from build123d import *

# Parameters (mm, degrees)
SKETCH1_W            = 40
SKETCH1_H            = 15
BOSS_EXTRUDE1_DEPTH  = 6
M3_CLEARANCE_HOLE1_D = 3.2
FILLET1_R            = 5


with BuildPart() as part:
    # Sketch1 → Boss-Extrude1 (new body)
    with BuildSketch(Plane(origin=(0, 0, 0), x_dir=(1, 0, 0), z_dir=(0, 1, 0))):
        Rectangle(SKETCH1_W, SKETCH1_H)
    extrude(amount=BOSS_EXTRUDE1_DEPTH)

    # M3 Clearance Hole1 (through all)
    with Locations(Plane(origin=(0, 6, 0), x_dir=(1, 0, 0), z_dir=(0, 1, 0))):
        with Locations((-15, 0), (15, 0)):
            Hole(M3_CLEARANCE_HOLE1_D / 2)

    # Fillet1
    fillet1_edges = [part.edges().sort_by_distance(p)[0] for p in [
        (20, 3, 7.5),
        (-20, 3, 7.5),
        (-20, 3, -7.5),
        (20, 3, -7.5),
    ]]
    fillet(fillet1_edges, radius=FILLET1_R)


solid = part.part
Verification items for the finished model (mm, model axes). Round coordinates to 2 decimals unless told otherwise and drop trailing zeros. Loops run counter-clockwise (first coordinate to the right, second up) from the corner with the lowest first, then second, coordinate; pieces in that order, holes last. Notation, with made-up numbers: (34, 11.5) - (66, 11.5) arc R9 cw to (66, 20.5) - close; hole circle Ø11 at (76, -31.5). An arc over 180 degrees is marked (long way). Use a Markdown table: item, result. Add a question column.
1. Gauge pin test, flat end, axial feed: pin 1 (1.5 mm diameter, centred on y = 4.5, z = -5.5, fed in from +X). Record the tip position at first contact, or that the pin passes through.
2. Section check B-B, the plane y = 1.4. Record the boundary of the cut face in (x, z), plus the area to 3 significant figures.
3. Release check for a two-part mould opening along Z. For faces 1 (the face through (16.6, 2.96, -0.07)), 2 (the face through (-13.4, 2.96, -0.07)), 3 (the face through (-18.57, 3.04, 6)), 4 (the face through (-20, 3, 0)) record: released by +Z, released by -Z, zero draft, split by the parting line, or undercut.
4. Section check A-A, the plane z = 0. Record the boundary of the cut face in (x, y), plus the area to 3 significant figures.
5. Thickness scan on probe 1 along Z at (x, y) = (15, 4.6); probe 2 along X at (y, z) = (2.9, 1); probe 3 along X at (y, z) = (2.55, 6.75). Record the ranges inside material, lowest first. Write a range as [from, to].
6. Section check C-C, the plane z = -5.25. Record the boundary of the cut face in (x, y), plus the area to 3 significant figures.
Checks:
| question | item | result |
|---|---|---|
| 1 | pin 1 | stops at x = 19.47 |
| 2 | outline | (-20, -2.5) arc R5 ccw to (-15, -7.5) - (15, -7.5) arc R5 ccw to (20, -2.5) - (20, 2.5) arc R5 ccw to (15, 7.5) - (-15, 7.5) arc R5 ccw to (-20, 2.5) - close; hole circle Ø3.2 at (-15, 0); hole circle Ø3.2 at (15, 0) |
| 2 | area | 562 mm^2 |
| 3 | face 1 | undercut |
| 3 | face 2 | undercut |
| 3 | face 3 | released by +Z |
| 3 | face 4 | zero draft |
| 4 | outline | (-20, 0) - (-16.6, 0) - (-16.6, 6) - (-20, 6) - close; (-13.4, 0) - (13.4, 0) - (13.4, 6) - (-13.4, 6) - close; (16.6, 0) - (20, 0) - (20, 6) - (16.6, 6) - close |
| 4 | area | 202 mm^2 |
| 5 | probe 1 | z = [-7.5, -1.6], [1.6, 7.5] |
| 5 | probe 2 | x = [-20, -16.25], [-13.75, 13.75], [16.25, 20] |
| 5 | probe 3 | x = [-17.63, 17.63] |
| 6 | outline | (-19.18, 0) - (19.18, 0) - (19.18, 6) - (-19.18, 6) - close |
| 6 | area | 230 mm^2 |
